Check sheet for the drawn part. Datum: minimum x, y, z corner. Units: mm. A direction names the side the tool comes from. Round coordinates to 2 decimals unless told otherwise and drop trailing zeros. Write each loop counter-clockwise with the first axis right and the second up, starting at its lowest first coordinate (ties: lowest second). Pieces come first, ordered by that corner, then holes. Notation, with made-up numbers: M 26.5,-31.75 L 49.5,-31.75 A24 cw 49.5,-8.75 Z; hole C 41,78 d9. An arc over 180 degrees is marked long. Put each result on its own line as item: value.
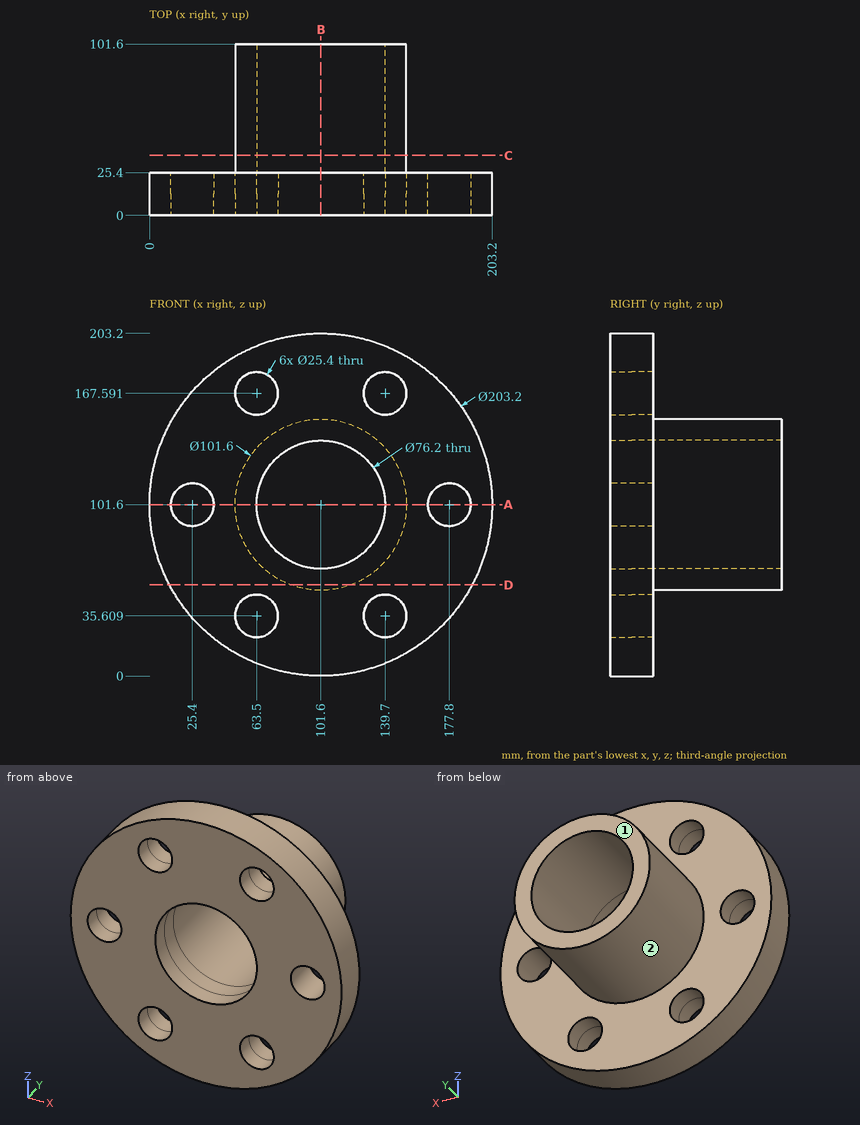
1. Access from +Z, -Z, +X, -X, +Y, -Y to the whole of each face (thin tool, end or side, straight path). Record for the marked faces 1 and 2.
Computed values:
face 1: +Z, -Z, +X, -X, +Y
face 2: +Y
2. Scan lines: probe 1 along X at (y, z) = (6, 101); probe 2 along X at (y, z) = (12.5, 44) (1 decimal); probe 3 along Z at (x, y) = (101, 9). Record each from-to range of solid material in increasing order.
Computed values:
probe 1: x = 0 to 12.71, 38.09 to 63.5, 139.7 to 165.11, 190.49 to 203.2
probe 2: x = 17.9 to 54, 73 to 130.2, 149.2 to 185.3
probe 3: z = 0 to 63.5, 139.7 to 203.2
3. Cross-section at A-A (z = 101.6). Enter the section's corners in (x, y).
Computed values:
outline: M 0,0 L 12.7,0 L 12.7,25.4 L 0,25.4 Z; M 38.1,0 L 63.5,0 L 63.5,101.6 L 50.8,101.6 L 50.8,25.4 L 38.1,25.4 Z; M 139.7,0 L 165.1,0 L 165.1,25.4 L 152.4,25.4 L 152.4,101.6 L 139.7,101.6 Z; M 190.5,0 L 203.2,0 L 203.2,25.4 L 190.5,25.4 Z
4. Cross-section at C-C (y = 35.5). Enter the section's corners in (x, z).
Computed values:
outline: C 101.6,101.6 d101.6; hole C 101.6,101.6 d76.2
5. Cross-section at B-B (x = 101.6). Enter the section's corners in (y, z), then the cut area to 3 significant figures.
Computed values:
outline: M 0,0 L 25.4,0 L 25.4,50.8 L 101.6,50.8 L 101.6,63.5 L 0,63.5 Z; M 0,139.7 L 101.6,139.7 L 101.6,152.4 L 25.4,152.4 L 25.4,203.2 L 0,203.2 Z
area: 5,160 mm2
6. Cross-section at D-D (z = 54). Enter the section's corners in (x, y) (1 decimal), then the cut area to 3 significant figures.
Computed values:
outline: M 11.8,0 L 191.4,0 L 191.4,25.4 L 119.3,25.4 L 119.3,101.6 L 83.9,101.6 L 83.9,25.4 L 11.8,25.4 Z
area: 7,260 mm2
7. Depth check by flat-ended pin: pin 1 Ø12 at (x, z) = (138.5, 152) entering from +Y; pin 2 Ø2 at (y, z) = (20.5, 73) entering from -X; pin 3 Ø10 at (x, y) = (181.5, 25) entering from +Z. Enter the tip coordinate at first touch or a pass-through.
Computed values:
pin 1: stops at y = 25.4
pin 2: stops at x = 3.82
pin 3: stops at z = 170.25
